Part model, mm, in its own coordinate system. Face numbers are marked on the shaded views. A direction names the side the tool comes from. Give positions to 0.01 mm unless a question says otherwise; leave off trailing zeros. Order: outer loops, then holes, each group sorted by start corner. A loop starts at its lowest first (then second) coordinate and runs counter-clockwise, first axis right, second up. Notation, with made-up numbers: M 36.5,14 L 84.5,14 A24 ccw 84.5,41 Z; hole C -38,12 d7. An arc over 180 degrees is marked long. Write each question's results on one line, items separated by ' | '. Start each with the question number.
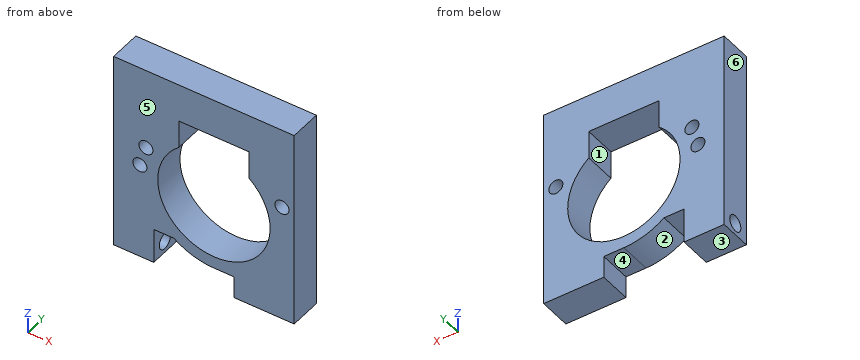
from build123d import *

# Parameters (mm, degrees)
SKETCH2_W                                 = 45
SKETCH2_H                                 = 50
STEPPER_SLIDER_BOSS_EXTRUDE1_DEPTH        = 8
SKETCH1_R                                 = 1.75
STEPPER_HOLE_CUT_EXTRUDE1_DEPTH           = 8
ADJUSTING_SCREW_POCKET_CUT_EXTRUDE1_DEPTH = 8
SKETCH4_R                                 = 2
ADJUSTING_SCREW_HOLE_CUT_EXTRUDE2_DEPTH   = 10


with BuildPart() as part:
    # Sketch2 → Stepper Slider Boss-Extrude1 (new body)
    with BuildSketch(Plane(origin=(0, 0, 0), x_dir=(1, 0, 0), z_dir=(0, 1, 0))):
        with Locations((-2.5, -2.5)):
            Rectangle(SKETCH2_W, SKETCH2_H)
    extrude(amount=-STEPPER_SLIDER_BOSS_EXTRUDE1_DEPTH)

    # Sketch1 → Stepper Hole Cut-Extrude1 (cut)
    with BuildSketch(Plane(origin=(0, 0, 0), x_dir=(1, 0, 0), z_dir=(0, 1, 0))):
        with Locations(Location((-18.45, -1.75, 0), (0, 0, 270))):
            Circle(SKETCH1_R)
        with Locations(Location((16.95, -7.041502622, 0), (0, 0, 270))):
            Circle(SKETCH1_R)
        with Locations(Location((-16.95, -7.041502622, 0), (0, 0, 270))):
            Circle(SKETCH1_R)
        with BuildLine():
            Line((8.75, -17.928746497), (8.75, -10.928746497))
            ThreePointArc((8.75, -10.928746497), (0, 14), (-8.75, -10.928746497))
            Line((-8.75, -10.928746497), (-8.75, -17.928746497))
            Line((-8.75, -17.928746497), (8.75, -17.928746497))
        make_face()
    extrude(amount=-STEPPER_HOLE_CUT_EXTRUDE1_DEPTH, mode=Mode.SUBTRACT)

    # Sketch3 → Adjusting Screw Pocket Cut-Extrude1 (cut)
    with BuildSketch(Plane(origin=(0, 0, 0), x_dir=(1, 0, 0), z_dir=(0, 1, 0))):
        with BuildLine():
            Line((0, 22.5), (-15, 22.5))
            Line((-15, 22.5), (-15, 13.747727085))
            Line((-15, 13.747727085), (-10, 13.747727085))
            ThreePointArc((-10, 13.747727085), (-5.257786585, 16.1664987), (0, 17))
            Line((0, 17), (5, 17))
            Line((5, 17), (5, 22.5))
            Line((5, 22.5), (0, 22.5))
        make_face()
    extrude(amount=-ADJUSTING_SCREW_POCKET_CUT_EXTRUDE1_DEPTH, mode=Mode.SUBTRACT)

    # Sketch4 → Adjusting Screw Hole Cut-Extrude2 (cut)
    with BuildSketch(Plane(origin=(-15, 0, 0), x_dir=(0, 0, -1), z_dir=(1, 0, 0))):
        with Locations((19.5, -4)):
            Circle(SKETCH4_R)
    extrude(amount=-ADJUSTING_SCREW_HOLE_CUT_EXTRUDE2_DEPTH, mode=Mode.SUBTRACT)


solid = part.part
(1) Saw through at A-A on y = -4. Give the cut face in (x, z), plus the area to 3 significant figures.
(2) Saw through at C-C on z = 14. Give the cut face in (x, y), plus the area to 3 significant figures.
(3) Probe L1, parallel to X at y = -6, z = -20; L2, parallel to X at y = -0.75, z = -3; L3, parallel to X at y = -1.5, z = 2.5. List the from-to ranges inside material, lowest first.
(4) Saw through at B-B on x = 16.95. Give the cut face in (y, z).
(5) Tool access for the marked faces 1, 2 and 3: list every direction of +Z, -Z, +X, -X, +Y, -Y with a clear straight run to the whole face (end or side of a thin tool).
(6) Pull direction X, two halves, no side cores. Call the marked faces 4, 5 and 6: +X half, -X half, draft (parallel to the pull), parting line (faces both ways), or undercut.
(7) Saw through at D-D on z = -19.5. Give the cut face in (x, y), plus the area to 3 significant figures.
(8) Drop flat-ended pins along their axis: P1, Ø3, axis at x = 16.95, z = 7.04, coming from the +Y side; P2, Ø2.5, axis at x = 4, y = -4.5, coming from the -Z side; P3, Ø2.5, axis at x = 3, y = -4, coming from the -Z side; P4, Ø3.5, axis at y = -4, z = -19.5, coming from the -X side. Give the stop position or say it passes through.
Taken from the geometry:
1) outline: M -25,-22.5 L -15,-22.5 L -15,-21.5 L -25,-21.5 Z; M -25,-17.5 L -15,-17.5 L -15,-13.75 L -10,-13.75 A17 ccw 0,-17 L 5,-17 L 5,-22.5 L 20,-22.5 L 20,27.5 L -25,27.5 Z; hole C -18.45,1.75 d3.5; hole C -16.95,7.04 d3.5; hole M -8.75,10.93 A14 ccw long 8.75,10.93 L 8.75,17.93 L -8.75,17.93 Z; hole C 16.95,7.04 d3.5 | area: 1,340 mm²
2) outline: M -25,-8 L -8.75,-8 L -8.75,0 L -25,0 Z; M 8.75,-8 L 20,-8 L 20,0 L 8.75,0 Z | area: 220 mm²
3) L1: x = -25 to -15, 5 to 20 | L2: x = -25 to -13.67, 13.67 to 20 | L3: x = -25 to -20.03, -16.87 to -13.77, 13.77 to 20
4) outline: M -8,-22.5 L 0,-22.5 L 0,5.29 L -8,5.29 Z; M -8,8.79 L 0,8.79 L 0,27.5 L -8,27.5 Z
5) face 1: +Y, -Y | face 2: -Z, +Y, -Y | face 3: -Z, +X, -X, +Y, -Y
6) face 4: undercut | face 5: draft | face 6: -X half
7) outline: M -25,-8 L -15,-8 L -15,-6 L -25,-6 Z; M -25,-2 L -15,-2 L -15,0 L -25,0 Z; M 5,-8 L 20,-8 L 20,0 L 5,0 Z | area: 160 mm²
8) P1: passes through | P2: stops at z = -22.5 | P3: stops at z = -17 | P4: stops at x = 5
